Build history of the part. All positions in model axes, mm. Round coordinates to 2 decimals unless told otherwise and drop trailing zeros. Loops run counter-clockwise (first coordinate to the right, second up) from the corner with the lowest first, then second, coordinate; pieces in that order, holes last. Notation, with made-up numbers: (77, 9.5) -> (83, 9.5) arc R26 ccw to (83, 23.5) -> close; hole circle Ø8 at (50, 80.25). An arc over 180 degrees is marked (long way). Put each result on its own line as item: value. Start each with the question number.
Item 1: Flat gauge pins, fed straight in: pin 1 Ø0.8 at (y, z) = (2, 164) entering from +X; pin 2 Ø2.5 at (x, z) = (0, 33.4) entering from +Y. Where does each tip first touch, or does it go through?
Item 2: Drill centre lines: probe 1 along Y at (x, z) = (-5, 89.5); probe 2 along X at (y, z) = (1.5, 66.5); probe 3 along X at (y, z) = (-1.6, 133.4). Where is each one in solid material? Low to high. Write a range as [from, to].
Item 3: Cut at A-A, the plane y = -2.5. Count the separate pieces of the cut face and the enclosed holes in it, plus the area to 3 significant figures.
Item 4: Cut at B-B, the plane z = 113.5. List the corners of the cut face in (x, y), plus the area to 3 significant figures.
```python
from build123d import *

# Parameters (mm, degrees)
SKETCH1_W           = 11.5
SKETCH1_H           = 7.8
BOSS_EXTRUDE1_DEPTH = 220
SKETCH2_W           = 0.835250229
SKETCH2_H           = 1.6
CUT_EXTRUDE1_DEPTH  = 221.109682886
SKETCH3_R           = 3
CUT_EXTRUDE2_DEPTH  = 4.7
SKETCH4_R           = 1.7
CUT_EXTRUDE3_DEPTH  = 221.125310903


with BuildPart() as part:
    # Sketch1 → Boss-Extrude1 (new body)
    with BuildSketch(Plane.XY):
        Rectangle(SKETCH1_W, SKETCH1_H)
    extrude(amount=BOSS_EXTRUDE1_DEPTH)

    # Sketch2 → Cut-Extrude1 (cut, through all)
    with BuildSketch(Plane.XY.offset(220)):
        with Locations((5.332374886, 1.7)):
            Rectangle(SKETCH2_W, SKETCH2_H)
        with Locations((-5.332374886, 1.7)):
            Rectangle(SKETCH2_W, SKETCH2_H)
    extrude(amount=-CUT_EXTRUDE1_DEPTH, mode=Mode.SUBTRACT)

    # Sketch3 → Cut-Extrude2 (cut)
    with BuildSketch(Plane(origin=(0, 3.9, 0), x_dir=(1, 0, 0), z_dir=(0, 1, 0))):
        with Locations(Location((0, -208.4, 0), (0, 0, 270))):
            Circle(SKETCH3_R)
        with Locations(Location((0, -183.4, 0), (0, 0, 270))):
            Circle(SKETCH3_R)
        with Locations(Location((0, -158.4, 0), (0, 0, 270))):
            Circle(SKETCH3_R)
        with Locations(Location((0, -133.4, 0), (0, 0, 270))):
            Circle(SKETCH3_R)
        with Locations(Location((0, -108.4, 0), (0, 0, 270))):
            Circle(SKETCH3_R)
        with Locations(Location((0, -83.4, 0), (0, 0, 270))):
            Circle(SKETCH3_R)
        with Locations(Location((0, -58.4, 0), (0, 0, 270))):
            Circle(SKETCH3_R)
        with Locations(Location((0, -33.4, 0), (0, 0, 270))):
            Circle(SKETCH3_R)
        with Locations(Location((0, -8.4, 0), (0, 0, 270))):
            Circle(SKETCH3_R)
        with Locations((0, 16.6)):
            Circle(SKETCH3_R)
        with Locations((0, 41.6)):
            Circle(SKETCH3_R)
        with Locations((0, 66.6)):
            Circle(SKETCH3_R)
        with Locations((0, 91.6)):
            Circle(SKETCH3_R)
        with Locations((0, 116.6)):
            Circle(SKETCH3_R)
        with Locations((0, 141.6)):
            Circle(SKETCH3_R)
        with Locations((0, 166.6)):
            Circle(SKETCH3_R)
        with Locations((0, 191.6)):
            Circle(SKETCH3_R)
        with Locations((0, 216.6)):
            Circle(SKETCH3_R)
        with Locations((0, 241.6)):
            Circle(SKETCH3_R)
        with Locations((0, 266.6)):
            Circle(SKETCH3_R)
        with Locations((0, 291.6)):
            Circle(SKETCH3_R)
        with Locations((0, 316.6)):
            Circle(SKETCH3_R)
        with Locations((0, 341.6)):
            Circle(SKETCH3_R)
        with Locations((0, 366.6)):
            Circle(SKETCH3_R)
        with Locations((0, 391.6)):
            Circle(SKETCH3_R)
        with Locations((0, 416.6)):
            Circle(SKETCH3_R)
        with Locations((0, 441.6)):
            Circle(SKETCH3_R)
        with Locations((0, 466.6)):
            Circle(SKETCH3_R)
        with Locations((0, 491.6)):
            Circle(SKETCH3_R)
        with Locations((0, 516.6)):
            Circle(SKETCH3_R)
    extrude(amount=-CUT_EXTRUDE2_DEPTH, mode=Mode.SUBTRACT)

    # Sketch4 → Cut-Extrude3 (cut, through all)
    with BuildSketch(Plane(origin=(0, -0.8, 0), x_dir=(1, 0, 0), z_dir=(0, 1, 0))):
        with Locations(Location((0, -208.4, 0), (0, 0, 270))):
            Circle(SKETCH4_R)
        with Locations(Location((0, -183.4, 0), (0, 0, 270))):
            Circle(SKETCH4_R)
        with Locations(Location((0, -158.4, 0), (0, 0, 270))):
            Circle(SKETCH4_R)
        with Locations(Location((0, -133.4, 0), (0, 0, 270))):
            Circle(SKETCH4_R)
        with Locations(Location((0, -108.4, 0), (0, 0, 270))):
            Circle(SKETCH4_R)
        with Locations(Location((0, -83.4, 0), (0, 0, 270))):
            Circle(SKETCH4_R)
        with Locations(Location((0, -58.4, 0), (0, 0, 270))):
            Circle(SKETCH4_R)
        with Locations(Location((0, -33.4, 0), (0, 0, 270))):
            Circle(SKETCH4_R)
        with Locations(Location((0, -8.4, 0), (0, 0, 270))):
            Circle(SKETCH4_R)
        with Locations((0, 16.6)):
            Circle(SKETCH4_R)
        with Locations((0, 41.6)):
            Circle(SKETCH4_R)
        with Locations((0, 66.6)):
            Circle(SKETCH4_R)
        with Locations((0, 91.6)):
            Circle(SKETCH4_R)
        with Locations((0, 116.6)):
            Circle(SKETCH4_R)
        with Locations((0, 141.6)):
            Circle(SKETCH4_R)
        with Locations((0, 166.6)):
            Circle(SKETCH4_R)
        with Locations((0, 191.6)):
            Circle(SKETCH4_R)
        with Locations((0, 216.6)):
            Circle(SKETCH4_R)
        with Locations((0, 241.6)):
            Circle(SKETCH4_R)
        with Locations((0, 266.6)):
            Circle(SKETCH4_R)
        with Locations((0, 291.6)):
            Circle(SKETCH4_R)
        with Locations((0, 316.6)):
            Circle(SKETCH4_R)
        with Locations((0, 341.6)):
            Circle(SKETCH4_R)
        with Locations((0, 366.6)):
            Circle(SKETCH4_R)
        with Locations((0, 391.6)):
            Circle(SKETCH4_R)
        with Locations((0, 416.6)):
            Circle(SKETCH4_R)
        with Locations((0, 441.6)):
            Circle(SKETCH4_R)
        with Locations((0, 466.6)):
            Circle(SKETCH4_R)
        with Locations((0, 491.6)):
            Circle(SKETCH4_R)
        with Locations((0, 516.6)):
            Circle(SKETCH4_R)
    extrude(amount=-CUT_EXTRUDE3_DEPTH, mode=Mode.SUBTRACT)


solid = part.part
```
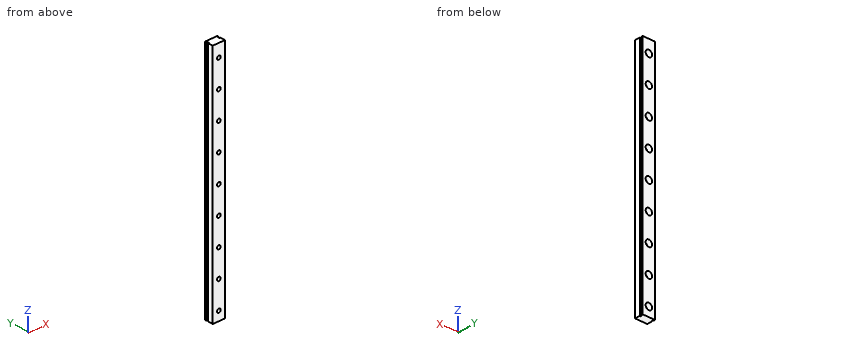
Reply:
1. pin 1: stops at x = 4.91
1. pin 2: passes through
2. probe 1: y = [-3.9, 0.9], [2.5, 3.9]
2. probe 2: x = [-4.91, 4.91]
2. probe 3: x = [-5.75, -1.7], [1.7, 5.75]
3. separate pieces: 1
3. enclosed holes: 9
3. area: 2,450 mm^2
4. outline: (-5.75, -3.9) -> (5.75, -3.9) -> (5.75, 0.9) -> (4.91, 0.9) -> (4.91, 2.5) -> (5.75, 2.5) -> (5.75, 3.9) -> (-5.75, 3.9) -> (-5.75, 2.5) -> (-4.91, 2.5) -> (-4.91, 0.9) -> (-5.75, 0.9) -> close
4. area: 87.0 mm^2
